```python
from build123d import *

# Parameters (mm, degrees)
F0_W     = 76.2
F0_H     = 38.1
F1_DEPTH = 25.4
F2_R     = 5.013158
F3_DEPTH = 25.4
F4_R     = 10.86406
F5_DEPTH = 38.1
F6_R     = 2.54
F7_W     = 18.654424
F7_H     = 24.483934


with BuildPart() as f1:
    # F0 (on Top) → F1 (new body)
    with BuildSketch(Plane.XY):
        Rectangle(F0_W, F0_H)
    extrude(amount=F1_DEPTH)

    # F2 (on Top) → F3 (cut)
    with BuildSketch(Plane.XY):
        with Locations((-30.48, -11.43)):
            Circle(F2_R)
        with Locations((30.48, -11.43)):
            Circle(F2_R)
        with Locations((30.48, 11.43)):
            Circle(F2_R)
        with Locations((-30.48, 11.43)):
            Circle(F2_R)
    extrude(amount=F3_DEPTH, mode=Mode.SUBTRACT)

    # F4 (on face) → F5 (join)
    with BuildSketch(Plane.XY.offset(25.4)):
        Circle(F4_R)
    extrude(amount=F5_DEPTH)

    # F6
    f6_edges = [f1.edges().sort_by_distance(p)[0] for p in [
        (0, 19.05, 25.4),
        (-38.1, 0, 25.4),
        (0, -19.05, 25.4),
        (38.1, 0, 25.4),
    ]]
    fillet(f6_edges, radius=F6_R)

    # F7 (on Front) → F8 (revolve, cut)
    with BuildSketch(Plane.XZ):
        with Locations((16.905574, 41.826721)):
            Rectangle(F7_W, F7_H)
    revolve(axis=Axis((0, 0, 25.4), (0, 0, -1)), mode=Mode.SUBTRACT)


solid = f1.part
```
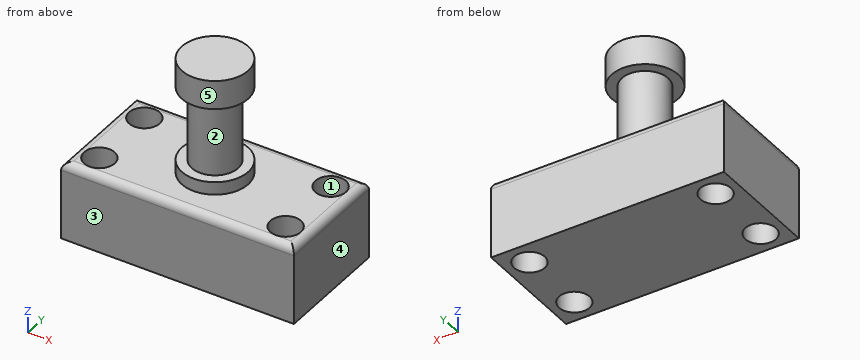
Geometry: final body of the model. Coordinates: model frame, mm. Face numbers are marked on the shaded views. A direction names the side the tool comes from. Give positions to 0.01 mm unless a question says otherwise; leave off trailing zeros. Loops run counter-clockwise (first coordinate to the right, second up) from the corner with the lowest first, then second, coordinate; pieces in that order, holes last. Notation, with made-up numbers: (50.25, 77) - (99.25, 77) arc R18 ccw to (99.25, 85) - close; hole circle Ø3 at (40.5, -35). An arc over 180 degrees is marked (long way). Answer as CSV lines item,"result". Start each with the question number.
(1) Section query D-D (x = 30). Output: boundary loops of the cut face in (y, z).
(2) Pin query (flat end, axial travel): P1, Ø8, axis at x = 26, y = 14, coming from the +Z side; P2, Ø6.5, axis at x = 3, y = 0, coming from the -Z side; P3, Ø9, axis at x = -30.48, y = 11.43, coming from the +Z side. Return the tip coordinate at first contact, or that it passes through.
(3) Section query A-A (x = -30.48). Output: boundary loops of the cut face in (y, z).
(4) Section query C-C (x = 12). Output: boundary loops of the cut face in (y, z), and give its area (3 significant figures).
(5) Section query B-B (y = 0). Output: boundary loops of the cut face in (x, z).
(6) Mould query, pull axis Y, two halves, no side actions, for the marked faces 1, 2 and 3. Classes: +Y half, -Y half, draft (parallel to the pull), parting line (faces both ways), or undercut.
(7) Ray query, line 1 along Y through (x, z) = (30.48, 16.25); line 2 along X through (y, z) = (-11, 10); line 3 along Z through (x, y) = (-15, 12.5). Return the intervals inside material, ascending. Write a range as [from, to].
(8) Reachability of the marked faces 4 and 5 from +Z, -Z, +X, -X, +Y, -Y: full face, straight path, thin tool, end or side. Return the list, or none.
Worked answers:
1,outline,"(-19.05, 0) - (-16.42, 0) - (-16.42, 25.4) - (-16.51, 25.4) arc R2.54 ccw to (-19.05, 22.86) - close; (-6.44, 0) - (6.44, 0) - (6.44, 25.4) - (-6.44, 25.4) - close; (16.42, 0) - (19.05, 0) - (19.05, 22.86) arc R2.54 ccw to (16.51, 25.4) - (16.42, 25.4) - close"
2,P1,"stops at z = 25.4"
2,P2,"stops at z = 0"
2,P3,"passes through"
3,outline,"(-19.05, 0) - (-16.44, 0) - (-16.44, 25.4) - (-16.51, 25.4) arc R2.54 ccw to (-19.05, 22.86) - close; (-6.42, 0) - (6.42, 0) - (6.42, 25.4) - (-6.42, 25.4) - close; (16.44, 0) - (19.05, 0) - (19.05, 22.86) arc R2.54 ccw to (16.51, 25.4) - (16.44, 25.4) - close"
4,outline,"(-19.05, 0) - (19.05, 0) - (19.05, 22.86) arc R2.54 ccw to (16.51, 25.4) - (-16.51, 25.4) arc R2.54 ccw to (-19.05, 22.86) - close"
4,area,"965 mm^2"
5,outline,"(-38.1, 0) - (38.1, 0) - (38.1, 22.86) arc R2.54 ccw to (35.56, 25.4) - (10.86, 25.4) - (10.86, 29.58) - (7.58, 29.58) - (7.58, 54.07) - (10.86, 54.07) - (10.86, 63.5) - (-10.86, 63.5) - (-10.86, 54.07) - (-7.58, 54.07) - (-7.58, 29.58) - (-10.86, 29.58) - (-10.86, 25.4) - (-35.56, 25.4) arc R2.54 ccw to (-38.1, 22.86) - close"
6,face 1,"undercut"
6,face 2,"parting line"
6,face 3,"-Y half"
7,line 1,"y = [-19.05, -16.44], [-6.42, 6.42], [16.44, 19.05]"
7,line 2,"x = [-38.1, -35.47], [-25.49, 25.49], [35.47, 38.1]"
7,line 3,"z = [0, 25.4]"
8,face 4,"+Z, -Z, +X, +Y, -Y"
8,face 5,"+Z"
